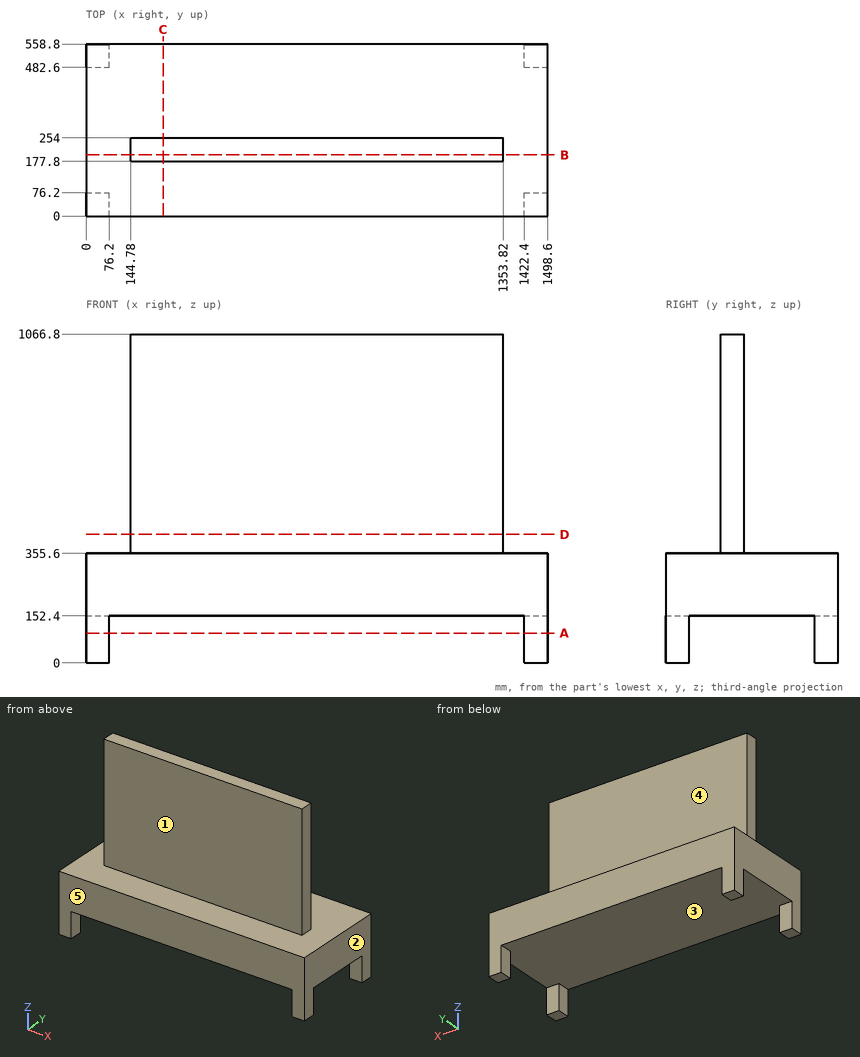
Job drawing, mm, ordinate dimensions from the low corner. One solid piece. A direction names the side the tool comes from. Give positions to 0.01 mm unless a question says otherwise; leave off trailing zeros. Order: outer loops, then holes, each group sorted by start corner. A loop starts at its lowest first (then second) coordinate and runs counter-clockwise, first axis right, second up. Notation, with made-up numbers: (89.25, -18) - (148.25, -18) arc R16 ccw to (148.25, 8) - close; hole circle Ø9 at (-15, -19). An arc over 180 degrees is marked (long way). Return JSON: item names as keys, results as strings.
1) Flat gauge pin, fed straight in: P1, Ø8, axis at x = 614, z = 382.5, coming from the +Y side. Where does the tip first touch, or does it go through?
Geometry says:
{"P1": "y = 254"}
2) Cut at D-D, the plane z = 417. Give the cut face in (x, y), plus the area to 3 significant figures.
Geometry says:
{"outline": "(144.78, 177.8) - (1353.82, 177.8) - (1353.82, 254) - (144.78, 254) - close", "area": "92,100 mm²"}
3) 3-axis set-ups, long thin cutter, end or side, ignore diameter. For the marked faces 4 and 5: which of +Z, -Z, +X, -X, +Y, -Y reach the whole face in a straight line?
Geometry says:
{"face 4": "+Z, +X, -X, +Y", "face 5": "+Z, -Z, +X, -X, -Y"}
4) Probe line 1 (Z direction, x = 461.5, y = 347); line 2 (Z direction, x = 200, y = 238.5); line 3 (Y direction, x = 698, z = 538.5). List the from-to ranges inside material, lowest first. Write a range as from..to.
Geometry says:
{"line 1": "152.4..355.6", "line 2": "152.4..1066.8", "line 3": "177.8..254"}
5) Cut at A-A, the plane z = 97. Give the cut face in (x, y), plus the area to 3 significant figures.
Geometry says:
{"outline": "(0, 0) - (76.2, 0) - (76.2, 76.2) - (0, 76.2) - close; (0, 482.6) - (76.2, 482.6) - (76.2, 558.8) - (0, 558.8) - close; (1422.4, 0) - (1498.6, 0) - (1498.6, 76.2) - (1422.4, 76.2) - close; (1422.4, 482.6) - (1498.6, 482.6) - (1498.6, 558.8) - (1422.4, 558.8) - close", "area": "23,200 mm²"}
6) Pull direction X, two halves, no side cores. Call the marked faces 1, 2 and 3: pulls with the +X half, pulls with the -X half, needs draft (parallel to the pull), parting line crosses it, or undercut.
Geometry says:
{"face 1": "needs draft", "face 2": "pulls with the +X half", "face 3": "undercut"}
7) Cut at C-C, the plane x = 250. Give the cut face in (y, z), plus the area to 3 significant figures.
Geometry says:
{"outline": "(0, 152.4) - (558.8, 152.4) - (558.8, 355.6) - (254, 355.6) - (254, 1066.8) - (177.8, 1066.8) - (177.8, 355.6) - (0, 355.6) - close", "area": "168,000 mm²"}
8) Cut at B-B, the plane y = 199. Give the cut face in (x, z), plus the area to 3 significant figures.
Geometry says:
{"outline": "(0, 152.4) - (1498.6, 152.4) - (1498.6, 355.6) - (1353.82, 355.6) - (1353.82, 1066.8) - (144.78, 1066.8) - (144.78, 355.6) - (0, 355.6) - close", "area": "1,160,000 mm²"}
